```python
from build123d import *

# Parameters (mm, degrees)
F6_R = 1


with BuildPart() as f3:
    # F0 (on Top) → F3 section 0
    with BuildSketch(Plane.XY, mode=Mode.PRIVATE) as f3_s0:
        Polygon((16.732227, 23.029935), (0, 53.037316), (-16.732227, 23.029935), (-50.441485, 16.389432), (-27.073313, -8.796653), (-31.174552, -42.90809), (0, -28.466566), (31.174552, -42.90809), (27.073313, -8.796653), (50.441485, 16.389432), align=None)
    loft([f3_s0.sketch, Vertex(0, 0, 12.7)])

    # F4: F3 across plane


with BuildPart() as f3_1:
    add(f3.part)
    add(f3.part.mirror(Plane.XY))

    # F7: sweep along a path in F5
    with BuildLine(Plane.XY) as f7_path:
        CenterArc((0, 56.037316), 3.75, 0, 360)
    # F6 (on Right) → F7 (sweep)
    with BuildSketch(Plane.YZ):
        with Locations((59.537316, 0)):
            Circle(F6_R)
    sweep(path=f7_path.line)


solid = f3_1.part
```
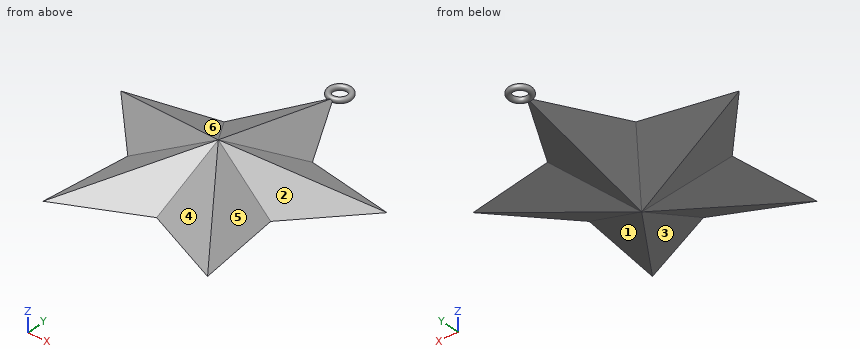
Verification items for the finished model (mm, model axes). Face numbers are marked on the shaded views. A direction names the side the tool comes from. Coordinates: 2 decimals unless noted, no trailing zeros. Order: outer loops, then holes, each group sorted by start corner. A loop starts at its lowest first (then second) coordinate and runs counter-clockwise, first axis right, second up. Notation, with made-up numbers: (-27.75, 52.5) - (-13.75, 52.5) arc R24 ccw to (-13.75, 82.5) - close; hole circle Ø1 at (-15, 23). An arc over 180 degrees is marked (long way). Return JSON: item names as keys, results as strings.
(1) Section check C-C, the plane x = 23.5. Record the cut outline in (y, z).
Filled sheet:
{"outline": "(-39.35, 0) - (-32.34, -3.13) - (-7.64, -1.68) - (7.64, -6.78) - (21.7, 0) - (7.64, 6.78) - (-7.64, 1.68) - (-32.34, 3.13) - close"}
(2) Go/stop test with flat-tipped pins: pin 1 (8 mm diameter, centred on x = -31, z = 5, fed in from +Y); pin 2 (3 mm diameter, centred on x = 5, y = 14, fed in from +Z); pin 3 (12 mm diameter, centred on x = -17.5, z = 2.5, fed in from -Y). Record where each tip stops, or that it passes through.
Filled sheet:
{"pin 1": "stops at y = 18.18", "pin 2": "stops at z = 7.94", "pin 3": "stops at y = -39.1"}
(3) Section check D-D, the plane y = 14.5. Record the cut outline in (x, z).
Filled sheet:
{"outline": "(-48.69, 0) - (-44.63, -1.46) - (-10.53, -4.7) - (0, -9.23) - (10.53, -4.7) - (44.63, -1.46) - (48.69, 0) - (44.63, 1.46) - (10.53, 4.7) - (0, 9.23) - (-10.53, 4.7) - (-44.63, 1.46) - close"}
(4) Mould release check, pull along Y, two halves, no side actions. Record for the marked faces 4, 5 and 6: pulls with the +Y half, pulls with the -Y half, needs draft (parallel to the pull), parting line crosses it, or undercut.
Filled sheet:
{"face 4": "pulls with the -Y half", "face 5": "undercut", "face 6": "pulls with the +Y half"}
(5) Section check B-B, the plane z = 8.5. Record the cut outline in (x, y), and give its area (3 significant figures).
Filled sheet:
{"outline": "(-16.68, 5.42) - (-8.95, -2.91) - (-10.31, -14.19) - (0, -9.41) - (10.31, -14.19) - (8.95, -2.91) - (16.68, 5.42) - (5.53, 7.62) - (0, 17.54) - (-5.53, 7.62) - close", "area": "485 mm^2"}
(6) Access from +Z, -Z, +X, -X, +Y, -Y to the whole of each face (thin tool, end or side, straight path). Record for the marked faces 1, 2 and 3.
Filled sheet:
{"face 1": "-Z, +X", "face 2": "+Z, +X", "face 3": "-Z, -Y"}
(7) Thickness scan on line 1 along Z through (x, y) = (-1, 6); line 2 along Z through (x, y) = (14, 14.5); line 3 along Y through (x, z) = (-16, -4.75). Record the ranges inside material, lowest first.
Filled sheet:
{"line 1": "z = -10.83 to 10.83", "line 2": "z = -4.37 to 4.37", "line 3": "y = -25.23 to 13.33"}
(8) Section check A-A, the plane y = -34. Record the cut outline in (x, z).
Filled sheet:
{"outline": "(-30.1, 0) - (-24.7, -2.64) - (-11.94, 0) - (-24.7, 2.64) - close; (11.94, 0) - (24.7, -2.64) - (30.1, 0) - (24.7, 2.64) - close"}
